Could you check a few things on this model? Use its own coordinates, in mm. Coordinates: 2 decimals unless noted, no trailing zeros. Loops run counter-clockwise (first coordinate to the right, second up) from the corner with the lowest first, then second, coordinate; pieces in that order, holes last.
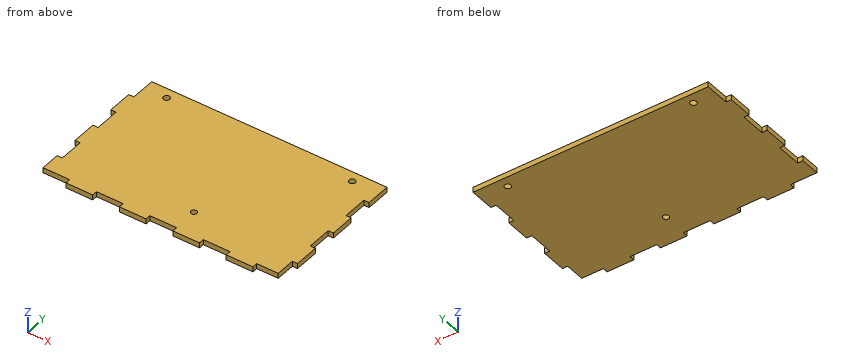
from build123d import *

# Parameters (mm, degrees)
SKETCH1_W                = 130
SKETCH1_H                = 80
BOSS_EXTRUDE1_DEPTH      = 2.8
SKETCH2_W                = 14.444444444
SKETCH2_H                = 2.8
SKETCH2_W_2              = 2.8
SKETCH2_H_2              = 13.333333334
SKETCH2_H_3              = 13.333333333
CUT_EXTRUDE1_DEPTH       = 153.669053839
CUT_EXTRUDE2_REACH       = 154.669
SKETCH3_R                = 1.7
TUNING_DRIVER_HOLE_REACH = 154.669
SKETCH4_R                = 1.6


with BuildPart() as part:
    # Sketch1 → Boss-Extrude1 (new body)
    with BuildSketch(Plane.XY):
        with Locations((65, 40)):
            Rectangle(SKETCH1_W, SKETCH1_H)
    extrude(amount=BOSS_EXTRUDE1_DEPTH)

    # Sketch2 → Cut-Extrude1 (cut, through all)
    with BuildSketch(Plane.XY.offset(2.8)):
        with Locations((7.222222222, 1.4)):
            Rectangle(SKETCH2_W, SKETCH2_H)
        with Locations((36.111111111, 1.4)):
            Rectangle(SKETCH2_W, SKETCH2_H)
        with Locations((65, 1.4)):
            Rectangle(SKETCH2_W, SKETCH2_H)
        with Locations((93.888888889, 1.4)):
            Rectangle(SKETCH2_W, SKETCH2_H)
        Polygon((115.555555556, 0), (115.555555556, 2.8), (127.2, 2.8), (127.2, 13.333333333), (130, 13.333333333), (130, 0), align=None)
        with Locations((1.4, 20)):
            Rectangle(SKETCH2_W_2, SKETCH2_H_2)
        with Locations((1.4, 46.666666667)):
            Rectangle(SKETCH2_W_2, SKETCH2_H_3)
        with Locations((1.4, 73.333333334)):
            Rectangle(SKETCH2_W_2, SKETCH2_H_3)
        with Locations((128.6, 33.333333334)):
            Rectangle(SKETCH2_W_2, SKETCH2_H_3)
        with Locations((128.6, 60)):
            Rectangle(SKETCH2_W_2, SKETCH2_H_2)
    extrude(amount=-CUT_EXTRUDE1_DEPTH, mode=Mode.SUBTRACT)

    # Sketch3 → Cut-Extrude2 (cut, up to next)
    with BuildSketch(Plane.XY.offset(2.8), mode=Mode.PRIVATE) as cut_extrude2_sk1:
        with Locations((14.8, 74.5)):
            Circle(SKETCH3_R)
    cut_extrude2_tool1 = extrude(cut_extrude2_sk1.sketch, amount=-CUT_EXTRUDE2_REACH, mode=Mode.PRIVATE) & part.part
    # Sketch3 → Cut-Extrude2 (cut, up to next)
    with BuildSketch(Plane.XY.offset(2.8), mode=Mode.PRIVATE) as cut_extrude2_sk2:
        with Locations(Location((115.2, 74.5, 0), (0, 0, 180))):
            Circle(SKETCH3_R)
    cut_extrude2_tool2 = extrude(cut_extrude2_sk2.sketch, amount=-CUT_EXTRUDE2_REACH, mode=Mode.PRIVATE) & part.part
    add(cut_extrude2_tool1.solids().sort_by_distance((14.8, 74.5, 2.8))[0], mode=Mode.SUBTRACT)
    add(cut_extrude2_tool2.solids().sort_by_distance((115.2, 74.5, 2.8))[0], mode=Mode.SUBTRACT)

    # Sketch4 → Tuning driver hole (cut, up to next)
    with BuildSketch(Plane(origin=(0, 0, 0), x_dir=(-1, 0, 0), z_dir=(0, 0, -1)), mode=Mode.PRIVATE) as tuning_driver_hole_sk1:
        with Locations((-71.91, 16.16)):
            Circle(SKETCH4_R)
    tuning_driver_hole_tool1 = extrude(tuning_driver_hole_sk1.sketch, amount=-TUNING_DRIVER_HOLE_REACH, mode=Mode.PRIVATE) & part.part
    add(tuning_driver_hole_tool1.solids().sort_by_distance((71.91, 16.16, 0))[0], mode=Mode.SUBTRACT)


solid = part.part
(1) Imagine slicing it at A-A, the plane y = 16.16. Write out the boundary of the cut face in (x, z).
Answers:
outline: (2.8, 0) - (70.31, 0) - (70.31, 2.8) - (2.8, 2.8) - close; (73.51, 0) - (130, 0) - (130, 2.8) - (73.51, 2.8) - close
(2) Imagine slicing it at D-D, the plane z = 1.6. State how many separate pieces and enclosed holes the cut face has, and give its area (3 significant figures).
Answers:
separate pieces: 1
enclosed holes: 3
area: 9,960 mm2
(3) Imagine slicing it at C-C, the plane x = 94.5. Write out the boundary of the cut face in (y, z).
Answers:
outline: (2.8, 0) - (80, 0) - (80, 2.8) - (2.8, 2.8) - close
(4) I need wall thicknesses on probe 1 along X at (y, z) = (74.5, 1.4); probe 2 along Y at (x, z) = (71.91, 1); probe 3 along Y at (x, z) = (14.8, 0.7). Which ranges of each line are inside material? Lowest first, please.
Answers:
probe 1: x = 2.8 to 13.1, 16.5 to 113.5, 116.9 to 130
probe 2: y = 2.8 to 14.56, 17.76 to 80
probe 3: y = 0 to 72.8, 76.2 to 80
(5) Imagine slicing it at B-B, the plane y = 74.5. Write out the boundary of the cut face in (x, z).
Answers:
outline: (2.8, 0) - (13.1, 0) - (13.1, 2.8) - (2.8, 2.8) - close; (16.5, 0) - (113.5, 0) - (113.5, 2.8) - (16.5, 2.8) - close; (116.9, 0) - (130, 0) - (130, 2.8) - (116.9, 2.8) - close
(6) For pin 1 (0.8 mm diameter, centred on x = 128.5, z = 2, fed in from -Y); pin 2 (1.4 mm diameter, centred on y = 22, z = 1, fed in from -X); pin 3 (1.4 mm diameter, centred on y = 0.5, z = 0.5, fed in from -X), each with a flat end and sliding along its axis, tell me the tip position at first contact or that it passes through.
Answers:
pin 1: stops at y = 13.33
pin 2: stops at x = 2.8
pin 3: stops at x = 14.44
